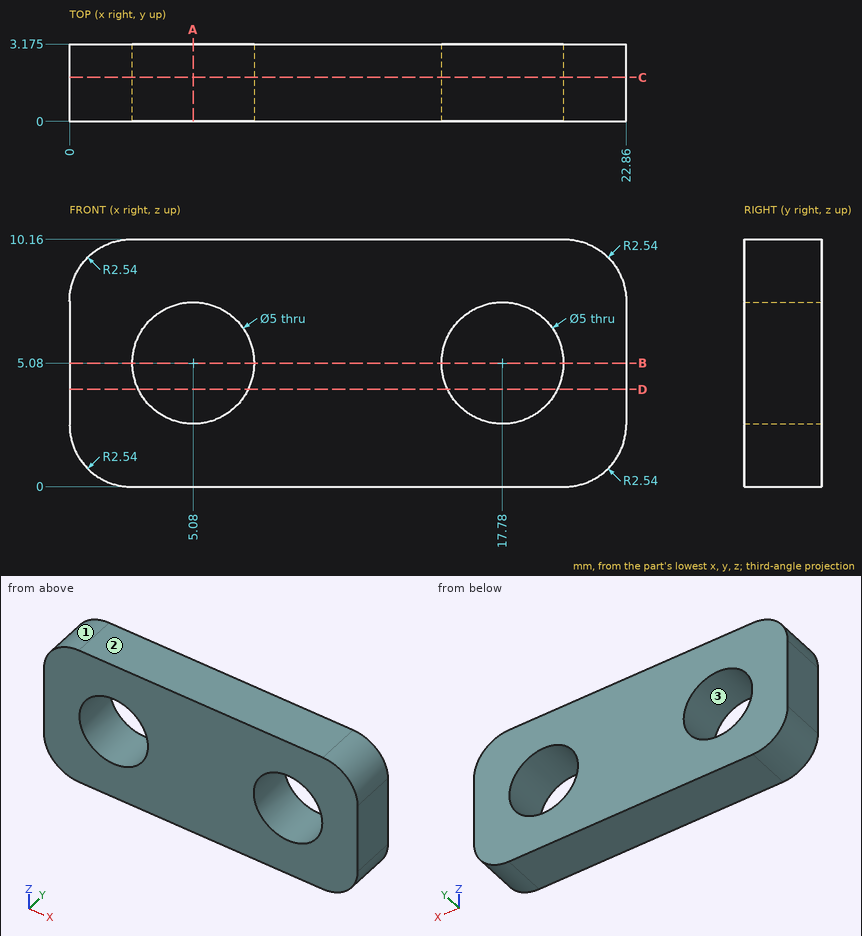
Geometry check sheet. Reference: drawing and pictorial views, mm from the part's lowest x, y, z. Give positions to 0.01 mm unless a question says otherwise; leave off trailing zeros. Order: outer loops, then holes, each group sorted by start corner. A loop starts at its lowest first (then second) coordinate and runs counter-clockwise, first axis right, second up. Notation, with made-up numbers: M 74.5,-25.5 L 114.5,-25.5 A18 cw 114.5,7.5 Z; hole C 42.5,-36.5 d11. An arc over 180 degrees is marked long. Return JSON: item names as keys, results as strings. Group by question number.
1) Scan lines: line 1 (X direction, y = 1.45, z = 5.08); line 2 (Z direction, x = 5.08, y = 1); line 3 (X direction, y = 2.45, z = 6.25). Record each from-to range of solid material in increasing order.
2) Section check B-B on z = 5.08. Record the cut outline in (x, y) (3 decimals), and give its area (3 significant figures).
3) Go/stop test with flat-tipped pins: pin 1 Ø1 at (y, z) = (2.5, 1) entering from +X; pin 2 Ø3 at (x, z) = (5.08, 5.08) entering from +Y. Record where each tip stops, or that it passes through.
4) Mould release check, pull along X, two halves, no side actions. Record for the marked faces 1, 2 and 3: pulls with the +X half, pulls with the -X half, needs draft (parallel to the pull), parting line crosses it, or undercut.
5) Section check C-C on y = 1.8. Record the cut outline in (x, z).
6) Section check D-D on z = 4. Record the cut outline in (x, y) (3 decimals), and give its area (3 significant figures).
7) Section check A-A on x = 5.08. Record the cut outline in (y, z) (3 decimals).
Answer block:
{
 "1": {"line 1": "x = 0 to 2.58, 7.58 to 15.28, 20.28 to 22.86", "line 2": "z = 0 to 2.58, 7.58 to 10.16", "line 3": "x = 0 to 2.87, 7.29 to 15.57, 19.99 to 22.86"},
 "2": {"outline": "M 0,0 L 2.58,0 L 2.58,3.175 L 0,3.175 Z; M 7.58,0 L 15.28,0 L 15.28,3.175 L 7.58,3.175 Z; M 20.28,0 L 22.86,0 L 22.86,3.175 L 20.28,3.175 Z", "area": "40.8 mm^2"},
 "3": {"pin 1": "stops at x = 22.64", "pin 2": "passes through"},
 "4": {"face 1": "pulls with the -X half", "face 2": "needs draft", "face 3": "undercut"},
 "5": {"outline": "M 0,2.54 A2.54 ccw 2.54,0 L 20.32,0 A2.54 ccw 22.86,2.54 L 22.86,7.62 A2.54 ccw 20.32,10.16 L 2.54,10.16 A2.54 ccw 0,7.62 Z; hole C 5.08,5.08 d5; hole C 17.78,5.08 d5"},
 "6": {"outline": "M 0,0 L 2.825,0 L 2.825,3.175 L 0,3.175 Z; M 7.335,0 L 15.525,0 L 15.525,3.175 L 7.335,3.175 Z; M 20.035,0 L 22.86,0 L 22.86,3.175 L 20.035,3.175 Z", "area": "43.9 mm^2"},
 "7": {"outline": "M 0,0 L 3.175,0 L 3.175,2.58 L 0,2.58 Z; M 0,7.58 L 3.175,7.58 L 3.175,10.16 L 0,10.16 Z"}
}
